Read the model definition and answer for the solid it produces. Units are mm, in the model's axes. A direction names the side the tool comes from. Round coordinates to 2 decimals unless told otherwise and drop trailing zeros. Loops run counter-clockwise (first coordinate to the right, second up) from the corner with the lowest first, then second, coordinate; pieces in that order, holes last. Notation, with made-up numbers: (1.5, -12) - (9.5, -12) arc R22 cw to (9.5, 5) - close; hole circle Ø7 at (79, 63.5). An arc over 180 degrees is marked (long way). Answer as CSV lines item,"result".
```python
from build123d import *

# Parameters (mm, degrees)
F0_W     = 180
F0_H     = 63
F1_DEPTH = 4
F2_R     = 27
F3_DEPTH = 4
F4_DEPTH = 247
F5_R     = 7.5
F6_DEPTH = 25
F7_T     = 1.5


# Not quite as in the source:
# - a shell that OpenCascade refuses in one call is made with other operations: the cavity is built on its own and cut out


with BuildPart() as f1:
    # F0 (on Front) → F1 (new body)
    with BuildSketch(Plane.XZ):
        with Locations((90, -31.5)):
            Rectangle(F0_W, F0_H)
    extrude(amount=F1_DEPTH)

    # F2 (on face) → F3 (join)
    with BuildSketch(Plane.XZ.offset(4)):
        with Locations((90, -31.5)):
            Circle(F2_R)
    extrude(amount=F3_DEPTH)

    # F2 (on face) → F4 (join)
    with BuildSketch(Plane.XZ.offset(4)):
        with BuildLine():
            ThreePointArc((37.5, -7.5), (35.3033008593, -2.1966991415), (30.0000000011, 0))
            ThreePointArc((30.0000000011, 0), (24.6966991407, -12.8033008585), (37.5, -7.5))
        make_face()
        with BuildLine():
            ThreePointArc((150, 0), (144.6966991411, -12.8033008589), (157.5, -7.5))
            ThreePointArc((157.5, -7.5), (155.3033008589, -2.1966991411), (150, 0))
        make_face()
    extrude(amount=F4_DEPTH)

    # F5 (on face) → F6 (cut)
    with BuildSketch(Plane.XZ.offset(8)):
        with Locations((90, -31.5)):
            Circle(F5_R)
    extrude(amount=-F6_DEPTH, mode=Mode.SUBTRACT)

    # F7: shell of thickness 1.5, made by hand


with BuildPart() as f7_core1:
    # F7_t2: copy of F1
    add(f1.part)

    # the walls: a layer under each face that stays
    f7_faces = [f7_core1.faces().sort_by_distance(p)[0] for p in [
        (90, -2, 0),
        (180, -2, -31.5),
        (0, -2, -31.5),
        (30, 0, -52.5),
        (30, -4, -52.5),
        (90, -2, -63),
        (82.5, -4, -31.5),
        (63, -6, -31.5),
        (29.9999999989, -127.5, -15),
        (150, -127.5, -15),
        (72, -8, -49.5),
    ]]
    thicken(f7_faces, amount=-F7_T, mode=Mode.SUBTRACT)

    # F7_s3 → F7_t4 (revolve, cut)
    with BuildSketch(Plane.XY.offset(-31.5)):
        Polygon((117.015, -4.015), (117, -2.5), (115.5, -2.5), (115.5, -4), align=None)
    revolve(axis=Axis((90, -4, -31.5), (0, -1, 0)), mode=Mode.SUBTRACT)

    # F7_s5 → F7_t6 (revolve, cut)
    with BuildSketch(Plane.YZ.offset(30)):
        Polygon((-4.015, 0.015), (-2.5, 0), (-2.5, -1.5), (-4, -1.5), align=None)
    revolve(axis=Axis((30, -4, -7.5), (0, -1, 0)), mode=Mode.SUBTRACT)

    # F7_s7 → F7_t8 (revolve, cut)
    with BuildSketch(Plane.YZ.offset(150)):
        Polygon((-4.015, 0.015), (-2.5, 0), (-2.5, -1.5), (-4, -1.5), align=None)
    revolve(axis=Axis((150, -4, -7.5), (0, -1, 0)), mode=Mode.SUBTRACT)


with BuildPart() as f1_1:
    add(f1.part)

    # what is left inside the walls is the cavity
    f7_cavity = [f7_core1.part.solids().sort_by_distance(p)[0] for p in [
        (90, -1.515, -41.5),
    ]]
    add(f7_cavity, mode=Mode.SUBTRACT)


solid = f1_1.part
```
1) A cutting plane is placed at B-B, the plane z = -49. Determine the outline of the cut face in (x, y).
Entries:
outline,"(0, -4) - (69.44, -4) - (69.44, -8) - (110.56, -8) - (110.56, -4) - (180, -4) - (180, 0) - (0, 0) - close; hole (1.5, -2.5) - (71.45, -2.5) - (71.45, -6.5) - (108.55, -6.5) - (108.55, -2.5) - (178.5, -2.5) - (178.5, -1.5) - (1.5, -1.5) - close"
2) A cutting plane is placed at A-A, the plane x = 90. Determine the outline of the cut face in (y, z), plus the area to 3 significant figures.
Entries:
outline,"(-8, -58.5) - (-4, -58.5) - (-4, -63) - (0, -63) - (0, -39) - (-8, -39) - close; (-8, -24) - (0, -24) - (0, 0) - (-4, 0) - (-4, -4.5) - (-8, -4.5) - close; hole (-6.5, -57) - (-2.5, -57) - (-2.5, -61.5) - (-1.5, -61.5) - (-1.5, -40.5) - (-6.5, -40.5) - close; hole (-6.5, -22.5) - (-1.5, -22.5) - (-1.5, -1.5) - (-2.5, -1.5) - (-2.5, -6) - (-6.5, -6) - close"
area,"174 mm^2"
3) A tool of negligible diameter and unlimited length cuts with its end or side. For faces 1 (the face through (96, -8, -37)), 2 (the face through (22.564, -125.771, -8.476)), 3 (the face through (101, -6.5, -31)), 4 (the face through (82.507, -4.056, -31.17)), from which of +Z, -Z, +X, -X, +Y, -Y can it reach the whole face along a straight path? Write none if from no direction.
Entries:
face 1,"+Z, -Z, -Y"
face 2,"-Y"
face 3,"none"
face 4,"+Y, -Y"
4) A cutting plane is placed at C-C, the plane y = -45. Determine the outline of the cut face in (x, z).
Entries:
outline,"circle Ø15 at (30, -7.5); circle Ø15 at (150, -7.5); hole circle Ø12 at (30, -7.5); hole circle Ø12 at (150, -7.5)"
5) Find the intervals of material crossed by line 1 (Z direction, x = 90, y = -3); line 2 (Z direction, x = 90, y = -4.75); line 3 (Y direction, x = 56, z = -26.5), in increasing order.
Entries:
line 1,"z = -63 to -57, -40.5 to -39, -24 to -22.5, -6 to 0"
line 2,"z = -58.5 to -57, -40.5 to -39, -24 to -22.5, -6 to -4.5"
line 3,"y = -4 to -2.5, -1.5 to 0"
6) A cutting plane is placed at D-D, the plane x = 127.5. Determine the outline of the cut face in (y, z).
Entries:
outline,"(-4, -63) - (0, -63) - (0, 0) - (-4, 0) - close; hole (-2.5, -61.5) - (-1.5, -61.5) - (-1.5, -1.5) - (-2.5, -1.5) - close"
7) The mould has two halves that part along Y. Classify faces 5 (the face through (104.515, -5.972, -8.733)), 6 (the face through (89, -4, -59)), 7 (the face through (89, -1.5, -18)): pulls with the +Y half, pulls with the -Y half, needs draft (parallel to the pull), parting line crosses it, or undercut.
Entries:
face 5,"needs draft"
face 6,"pulls with the -Y half"
face 7,"undercut"
8) Each of these flat-tipped pins is pushed along its axis until it touches: P1, Ø0.5, axis at y = -2, z = -17.5, coming from the -X side; P2, Ø1, axis at x = 99, z = -12.5, coming from the -Y side; P3, Ø4, axis at y = -130.5, z = -7, coming from the -X side; P4, Ø11, axis at x = 30, z = -7.5, coming from the -Y side. Where does it stop, or does it pass through?
Entries:
P1,"stops at x = 0"
P2,"stops at y = -8"
P3,"stops at x = 22.5"
P4,"stops at y = -1.5"
